Read the model definition and answer for the solid it produces. Units are mm, in the model's axes. A direction names the side the tool comes from. Round coordinates to 2 decimals unless told otherwise and drop trailing zeros. Order: outer loops, then holes, each group sorted by start corner. A loop starts at its lowest first (then second) coordinate and runs counter-clockwise, first axis right, second up. Notation, with made-up numbers: (20, -20) -> (41, -20) arc R22 ccw to (41, -10) -> close; hole circle Ø6 at (84, 85.25). An arc over 180 degrees is marked (long way). One line per item, written item: value. Start each with the question number.
1. The mould has two halves that part along Z. Classify faces 4 (the face through (0, 38, 2.54)), 5 (the face through (-1, 38, 0)), 6 (the face through (-0.978, 60.316, 120.739)): released by +Z, released by -Z, zero draft, split by the parting line, or undercut.
2. Section B-B (z = 116.5) is taken. Give the vertices of the cut face in (x, y).
3. Consider line 1 (X direction, y = 38.1, z = 32); line 2 (X direction, y = 38.1, z = 119); line 3 (Z direction, x = -21, y = 44.5). Determine where each line is inside the solid, lowest interval first.
4. Section D-D (z = 71) is taken. Give the vertices of the cut face in (x, y), then the cut area to 3 significant figures.
5. Section A-A (y = 38.1) is taken. Give the vertices of the cut face in (x, z), then the cut area to 3 significant figures.
6. For faces 1 (the face through (-5.917, 19.312, 120.137)), 2 (the face through (34.714, 45.809, 52.145)), 3 (the face through (23.183, 68.335, 51.511)), determine the directions among +Z, -Z, +X, -X, +Y, -Y from which every point of the face is accessible in a straight line to the end or side of a thin tool.
7. Section C-C (x = 0) is taken. Give the vertices of the cut face in (y, z).
8. Flat-ended cylindrical pins translate along their axes: pin 1 Ø3 at (y, z) = (18.5, 96) entering from -X; pin 2 Ø2 at (y, z) = (44.5, 109.5) entering from -X; pin 3 Ø5 at (x, z) = (-1, 33) entering from +Y; pin 4 Ø6 at (x, z) = (23, 91.5) entering from +Y. Find the tip coordinate at first contact, or state that the pin passes through.
from build123d import *

# Parameters (mm, degrees)
SHELL1_T = -2.54


with BuildPart() as part:
    # Sketch1 → Revolve1 (revolve)
    with BuildSketch(Plane.YZ):
        Polygon((0, 0), (0, 101.6), (15.862294916, 114.3), (15.862294916, 127), (38.1, 127), (38.1, 0), align=None)
    revolve(axis=Axis((0, 38.1, 127), (0, 0, -1)))

    # Shell1
    shell1_openings = [part.faces().sort_by_distance(p)[0] for p in [
        (0, 38.1, 127),
    ]]
    offset(amount=SHELL1_T, openings=shell1_openings, kind=Kind.INTERSECTION)


solid = part.part
Answer:
1. face 4: undercut
1. face 5: released by -Z
1. face 6: zero draft
2. outline: circle Ø44.48 at (0, 38.1); hole circle Ø39.4 at (0, 38.1)
3. line 1: -38.1 to -35.56, 35.56 to 38.1
3. line 2: -22.24 to -19.7, 19.7 to 22.24
3. line 3: 0 to 2.54, 111.27 to 127
4. outline: circle Ø76.2 at (0, 38.1); hole circle Ø71.12 at (0, 38.1)
4. area: 588 mm^2
5. outline: (-38.1, 0) -> (38.1, 0) -> (38.1, 101.6) -> (22.24, 114.3) -> (22.24, 127) -> (19.7, 127) -> (19.7, 113.08) -> (35.56, 100.38) -> (35.56, 2.54) -> (-35.56, 2.54) -> (-35.56, 100.38) -> (-19.7, 113.08) -> (-19.7, 127) -> (-22.24, 127) -> (-22.24, 114.3) -> (-38.1, 101.6) -> close
5. area: 865 mm^2
6. face 1: +Z
6. face 2: none
6. face 3: +Z, -Z
7. outline: (0, 0) -> (76.2, 0) -> (76.2, 101.6) -> (60.34, 114.3) -> (60.34, 127) -> (57.8, 127) -> (57.8, 113.08) -> (73.66, 100.38) -> (73.66, 2.54) -> (2.54, 2.54) -> (2.54, 100.38) -> (18.4, 113.08) -> (18.4, 127) -> (15.86, 127) -> (15.86, 114.3) -> (0, 101.6) -> close
8. pin 1: x = -33.53
8. pin 2: x = -28.8
8. pin 3: y = 76.2
8. pin 4: y = 70.53
